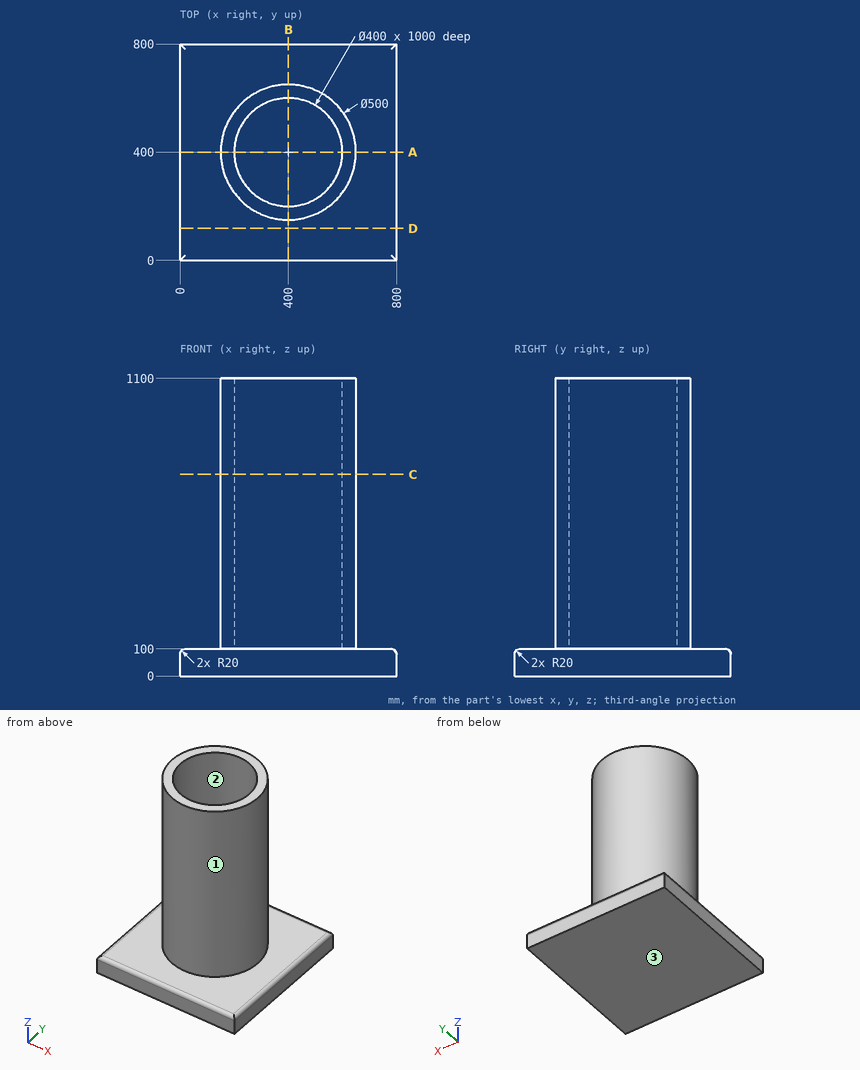
Part print with two shaded views. Sizes in mm from the minimum x, y, z corner. Round coordinates to 2 decimals unless told otherwise and drop trailing zeros. Order: outer loops, then holes, each group sorted by start corner. A loop starts at its lowest first (then second) coordinate and runs counter-clockwise, first axis right, second up. Notation, with made-up numbers: (18.5, 39.25) - (48.5, 39.25) arc R22 cw to (48.5, 68.25) - close; hole circle Ø6 at (78, -32). An arc over 180 degrees is marked (long way). Answer as CSV lines item,"result". Start each with the question number.
1. Drill centre lines: L1, parallel to Y at x = 390.5, z = 390.5; L2, parallel to Y at x = 400, z = 491.5; L3, parallel to X at y = 394.5, z = 230. Where is each one in solid material? Low to high. Write a range as [from, to].
2. Saw through at A-A, the plane y = 400. Write the cut outline in (x, z), and give its area (3 significant figures).
3. Pull direction Y, two halves, no side cores. Call the marked faces 1, 2 and 3: +Y half, -Y half, draft (parallel to the pull), parting line (faces both ways), or undercut.
4. Pin check, flat tips, straight feed: pin 1 (1 mm diameter, centred on y = 486.5, z = 862.5, fed in from -X); pin 2 (2 mm diameter, centred on x = 590, z = 568, fed in from +Y); pin 3 (2 mm diameter, centred on y = 603, z = 782.5, fed in from -X). Stop position of each tip, or through.
5. Saw through at D-D, the plane y = 118. Write the cut outline in (x, z).
6. Saw through at C-C, the plane z = 745.5. Write the cut outline in (x, y).
Model answer:
1,L1,"y = [150.18, 200.23], [599.77, 649.82]"
1,L2,"y = [150, 200], [600, 650]"
1,L3,"x = [150.06, 200.08], [599.92, 649.94]"
2,outline,"(0, 0) - (800, 0) - (800, 80) arc R20 ccw to (780, 100) - (650, 100) - (650, 1100) - (600, 1100) - (600, 100) - (200, 100) - (200, 1100) - (150, 1100) - (150, 100) - (20, 100) arc R20 ccw to (0, 80) - close"
2,area,"180,000 mm²"
3,face 1,"parting line"
3,face 2,"undercut"
3,face 3,"draft"
4,pin 1,"stops at x = 165.26"
4,pin 2,"stops at y = 563.64"
4,pin 3,"stops at x = 252.7"
5,outline,"(0, 0) - (800, 0) - (800, 80) arc R20 ccw to (780, 100) - (20, 100) arc R20 ccw to (0, 80) - close"
6,outline,"circle Ø500 at (400, 400); hole circle Ø400 at (400, 400)"
